Read the model definition and answer for the solid it produces. Units are mm, in the model's axes. Face numbers are marked on the shaded views. A direction names the side the tool comes from. Coordinates: 2 decimals unless noted, no trailing zeros. Order: outer loops, then holes, each group sorted by start corner. A loop starts at its lowest first (then second) coordinate and runs counter-clockwise, first axis right, second up. Notation, with made-up numbers: (-25.5, -36) -> (10.5, -36) arc R24 ccw to (10.5, -2) -> close; hole circle Ø11 at (-37, 57.5). An arc over 180 degrees is marked (long way). Answer in a Markdown table with one row per item.
from build123d import *

# Parameters (mm, degrees)
SKETCH1_W           = 76.2
SKETCH1_H           = 50.8
BOSS_EXTRUDE1_DEPTH = 12.7
BOSS_EXTRUDE1_TAPER = 3
SKETCH2_W           = 95.25
SKETCH2_H           = 69.85
BOSS_EXTRUDE2_DEPTH = 3.175
SKETCH3_W           = 95.25
SKETCH3_H           = 69.85
SKETCH3_W_2         = 88.9
SKETCH3_H_2         = 63.5
BOSS_EXTRUDE3_DEPTH = 15.875
DRAFT1_ANGLE        = 3
SKETCH4_W           = 68.518842406
SKETCH4_H           = 43.118842406
CUT_EXTRUDE1_DEPTH  = 3.175
CUT_EXTRUDE1_DRAFT  = -3
SKETCH6_R           = 12.7
SKETCH6_R_2         = 9.525
BOSS_EXTRUDE5_DEPTH = 3.175
BOSS_EXTRUDE6_REACH = 108.018
CIRPATTERN1_COUNT   = 8
DRAFT2_ANGLE        = 3


with BuildPart() as part:
    # Sketch1 → Boss-Extrude1 (new body)
    with BuildSketch(Plane(origin=(0, 0, 0), x_dir=(1, 0, 0), z_dir=(0, 1, 0))):
        with Locations((38.1, 25.4)):
            Rectangle(SKETCH1_W, SKETCH1_H)
    extrude(amount=BOSS_EXTRUDE1_DEPTH, taper=BOSS_EXTRUDE1_TAPER)

    # Sketch2 → Boss-Extrude2 (add)
    with BuildSketch(Plane.XZ):
        with Locations((38.1, -25.4)):
            Rectangle(SKETCH2_W, SKETCH2_H)
    extrude(amount=BOSS_EXTRUDE2_DEPTH)

    # Sketch3 → Boss-Extrude3 (add)
    with BuildSketch(Plane(origin=(0, 0, 0), x_dir=(1, 0, 0), z_dir=(0, 1, 0))):
        with Locations((38.1, 25.4)):
            Rectangle(SKETCH3_W, SKETCH3_H)
        with Locations((38.1, 25.4)):
            Rectangle(SKETCH3_W_2, SKETCH3_H_2, mode=Mode.SUBTRACT)
    extrude(amount=BOSS_EXTRUDE3_DEPTH)

    # Draft1
    draft1_faces = [part.faces().sort_by_distance(p)[0] for p in [
        (82.55, 7.9375, -25.4),
        (38.1, 7.9375, -57.15),
        (38.1, 7.9375, 6.35),
        (-6.35, 7.9375, -25.4),
    ]]
    draft(draft1_faces, Plane.ZX, DRAFT1_ANGLE)


with BuildPart() as cut_extrude1_tool:
    # Sketch4 → Cut-Extrude1 (with draft: the straight prism first)
    with BuildSketch(Plane(origin=(0, 12.7, 0), x_dir=(1, 0, 0), z_dir=(0, 1, 0))):
        with Locations((38.1, 25.4)):
            Rectangle(SKETCH4_W, SKETCH4_H)
    extrude(amount=-CUT_EXTRUDE1_DEPTH)
    # Cut-Extrude1: the draft: its side faces are tilted about the plane it starts from
    cut_extrude1_sides = [cut_extrude1_tool.faces().sort_by_distance(p)[0] for p in [
        (3.840578797, 11.1125, -25.4),
        (38.1, 11.1125, -3.840578797),
        (72.359421203, 11.1125, -25.4),
        (38.1, 11.1125, -46.959421203),
    ]]
    draft(cut_extrude1_sides, Plane(origin=(0, 12.7, 0), x_dir=(1, 0, 0), z_dir=(0, 1, 0)), CUT_EXTRUDE1_DRAFT)


with BuildPart() as part_1:
    add(part.part)

    # Cut-Extrude1: cut by cut_extrude1_tool
    add(cut_extrude1_tool.part, mode=Mode.SUBTRACT)

    # Sketch6 → Boss-Extrude5 (add)
    with BuildSketch(Plane(origin=(0, 9.525, 0), x_dir=(1, 0, 0), z_dir=(0, 1, 0))):
        with Locations(Location((38.1, 25.4, 0), (0, 0, 90))):
            Circle(SKETCH6_R)
        with Locations(Location((38.1, 25.4, 0), (0, 0, 90))):
            Circle(SKETCH6_R_2, mode=Mode.SUBTRACT)
    extrude(amount=BOSS_EXTRUDE5_DEPTH)

    # Sketch7 → Boss-Extrude6 (add, up to next)
    with BuildSketch(Plane(origin=(0, 12.7, 0), x_dir=(1, 0, 0), z_dir=(0, 1, 0)), mode=Mode.PRIVATE) as boss_extrude6_sk1:
        with BuildLine():
            Line((42.624193754, 40.616678214), (40.51523203, 37.868225786))
            ThreePointArc((40.51523203, 37.868225786), (42.960079591, 37.133270063), (45.208540056, 35.924193949))
            Line((45.208540056, 35.924193949), (45.66072827, 39.358904435))
            ThreePointArc((45.66072827, 39.358904435), (44.175099489, 40.066587579), (42.624193754, 40.616678214))
        make_face()
    boss_extrude6_tool1 = extrude(boss_extrude6_sk1.sketch, amount=-BOSS_EXTRUDE6_REACH, mode=Mode.PRIVATE) - part_1.part
    boss_extrude6 = boss_extrude6_tool1.solids().sort_by_distance((43.502556, 12.7, -38.442924))[0]
    add(boss_extrude6)

    # CirPattern1: Boss-Extrude6 ×8 about axis
    cirpattern1_axis = Axis((38.1, 0, -25.4), (0, 1, 0))
    for i in range(1, CIRPATTERN1_COUNT):
        add(boss_extrude6.rotate(cirpattern1_axis, i * 360 / CIRPATTERN1_COUNT))

    # Draft2
    draft2_faces = [part_1.faces().sort_by_distance(p)[0] for p in [
        (30.765365837, 11.1125, -37.641549192),
        (32.024900511, 11.1125, -40.066587579),
        (34.630287108, 11.1125, -39.242452),
        (50.8, 11.1125, -25.4),
        (38.1, 11.1125, -15.875),
        (47.080256121, 11.1125, -34.380256121),
        (45.434634163, 11.1125, -37.641549192),
        (44.175099489, 11.1125, -40.066587579),
        (41.569712892, 11.1125, -39.242452),
        (38.1, 11.1125, -38.1),
        (51.942452, 11.1125, -28.869712892),
        (52.766587579, 11.1125, -31.475099489),
        (50.341549192, 11.1125, -32.734634163),
        (47.080256121, 11.1125, -16.419743879),
        (50.341549192, 11.1125, -18.065365837),
        (41.569712892, 11.1125, -11.557548),
        (52.766587579, 11.1125, -19.324900511),
        (51.942452, 11.1125, -21.930287108),
        (38.1, 11.1125, -12.7),
        (44.175099489, 11.1125, -10.733412421),
        (45.434634163, 11.1125, -13.158450808),
        (29.119743879, 11.1125, -16.419743879),
        (30.765365837, 11.1125, -13.158450808),
        (32.024900511, 11.1125, -10.733412421),
        (34.630287108, 11.1125, -11.557548),
        (25.4, 11.1125, -25.4),
        (24.257548, 11.1125, -21.930287108),
        (23.433412421, 11.1125, -19.324900511),
        (25.858450808, 11.1125, -18.065365837),
        (29.119743879, 11.1125, -34.380256121),
        (25.858450808, 11.1125, -32.734634163),
        (23.433412421, 11.1125, -31.475099489),
        (24.257548, 11.1125, -28.869712892),
    ]]
    draft(draft2_faces, Plane.ZX.offset(9.525), DRAFT2_ANGLE)


solid = part_1.part
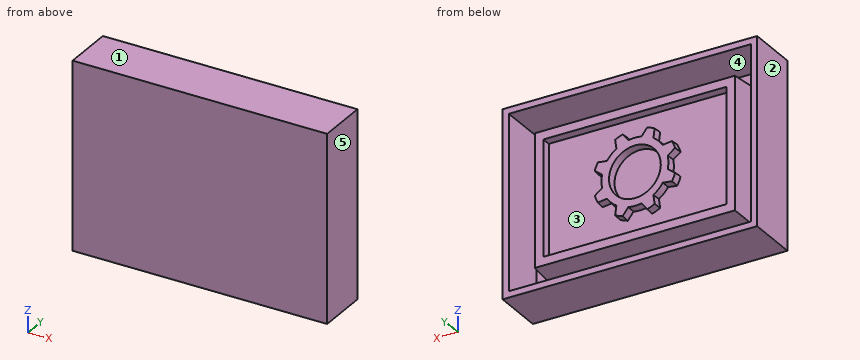
Q1. For the marked faces 4 and 5, determine the directions among +Z, -Z, +X, -X, +Y, -Y from which every point of the face is accessible in a straight line to the end or side of a thin tool.
Outcome:
| item | result |
|---|---|
| face 4 | +Y |
| face 5 | +Z, -Z, +X, +Y, -Y |
Q2. For a pull along X with two mould halves and no side action, classify the marked faces 1, 2 and 3 as pulls with the +X half, pulls with the -X half, needs draft (parallel to the pull), parting line crosses it, or undercut.
Outcome:
| item | result |
|---|---|
| face 1 | needs draft |
| face 2 | pulls with the -X half |
| face 3 | undercut |
Q3. Consider line 1 (Z direction, x = -5.5, y = 0.25) (3 decimals); line 2 (Z direction, x = 69, y = 3.75) (3 decimals); line 3 (Z direction, x = 39.5, y = 11.5) (3 decimals). Determine where each line is inside the solid, lowest interval first.
Outcome:
| item | result |
|---|---|
| line 1 | -60.325 to -57.163, 6.363 to 9.525 |
| line 2 | -60.325 to -57.347, -50.603 to -0.197, 6.547 to 9.525 |
| line 3 | -60.325 to -57.753, -50.197 to -46.897, -37.918 to -34.926, -15.874 to -12.882, -3.903 to -0.603, 6.953 to 9.525 |
Q4. The part is cut by section A-A (z = 1.5). Write down the section's boundary in (x, y) (3 decimals), then the cut area to 3 significant figures.
Outcome:
| item | result |
|---|---|
| outline | (-9.525, -3.175) -> (85.725, -3.175) -> (85.725, 15.875) -> (83.382, 15.875) -> (82.55, 0) -> (-6.35, 0) -> (-7.182, 15.875) -> (-9.525, 15.875) -> close |
| area | 390 mm² |
Q5. Given pin 1 (15 mm diameter, centred on x = 34.5, z = -29, fed in from +Y), flat-ended and moving along its own axis, determine where the tip first touches the part or whether it passes through.
Outcome:
| item | result |
|---|---|
| pin 1 | y = 12.7 |
Q6. The part is cut by section B-B (y = 8.5). Give the number of separate pieces and of enclosed holes in the cut face, then the cut area to 3 significant figures.
Outcome:
| item | result |
|---|---|
| separate pieces | 2 |
| enclosed holes | 1 |
| area | 4,630 mm² |
